Print and shaded views of the part. All mm, measured from the part's lowest x, y and z. Round coordinates to 2 decimals unless told otherwise and drop trailing zeros. Loops run counter-clockwise (first coordinate to the right, second up) from the corner with the lowest first, then second, coordinate; pieces in that order, holes last. Notation, with made-up numbers: (0.25, 46) - (59.25, 46) arc R27 cw to (59.25, 68) - close; hole circle Ø10 at (81.5, 36.5). An arc over 180 degrees is marked (long way). Use one line per item in the form item = value. Start each with the question number.
Q1. Saw through at A-A (z = 2.7). Give the cut face in (x, y), then the cut area to 3 significant figures.
Q2. Saw through at D-D (y = 4). Give the cut face in (x, z).
Q3. Saw through at B-B (x = 15.25). Give the cut face in (y, z).
Q4. Mould opens along X. For the marked faces 1 and 2 say: released by +X, released by -X, zero draft, split by the parting line, or undercut.
Q5. Saw through at C-C (y = 16). Give the cut face in (x, z), then the cut area to 3 significant figures.
Q6. Drill centre lines: line 1 (X direction, y = 10.25, z = 3.4); line 2 (X direction, y = 14, z = 1.05); line 3 (Y direction, x = 9, z = 0.5). Where is each one in solid material? Low to high.
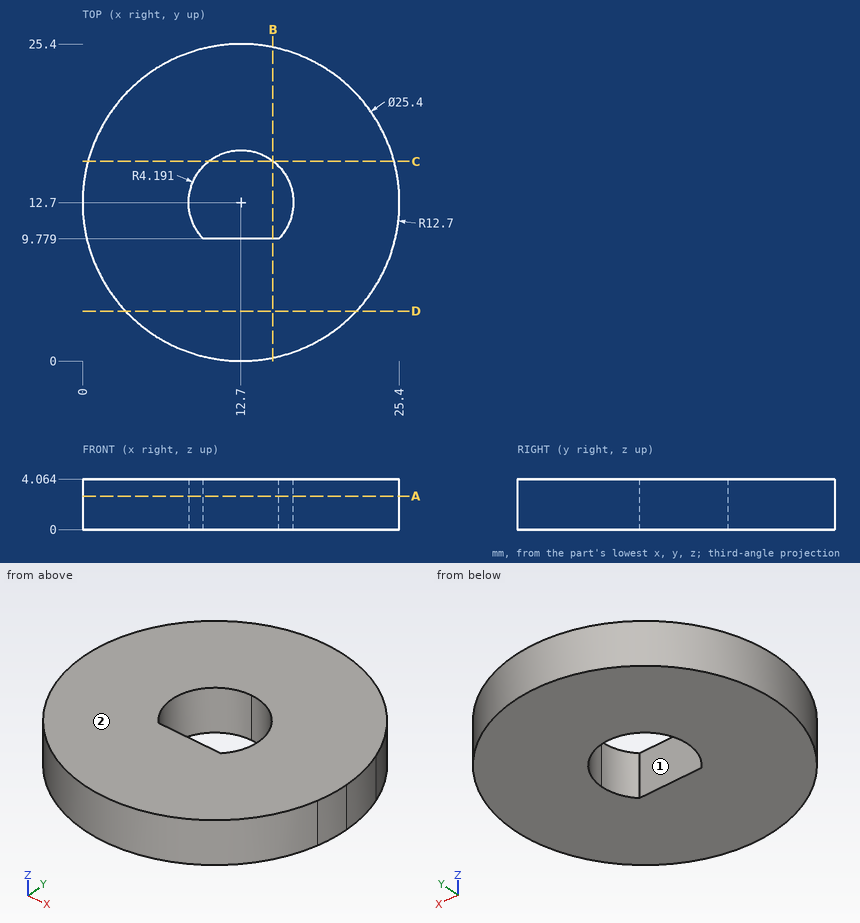
Report:
q1.outline = circle Ø25.4 at (12.7, 12.7); hole (9.69, 9.78) - (15.71, 9.78) arc R4.19 ccw (long way) to start
q1.area = 457 mm²
q2.outline = (3.45, 0) - (21.95, 0) - (21.95, 4.06) - (3.45, 4.06) - close
q3.outline = (0.26, 0) - (9.78, 0) - (9.78, 4.06) - (0.26, 4.06) - close; (16.03, 0) - (25.14, 0) - (25.14, 4.06) - (16.03, 4.06) - close
q4.face_1 = undercut
q4.face_2 = zero draft
q5.outline = (0.44, 0) - (10.12, 0) - (10.12, 4.06) - (0.44, 4.06) - close; (15.28, 0) - (24.96, 0) - (24.96, 4.06) - (15.28, 4.06) - close
q5.area = 78.7 mm²
q6.line_1 = 0.24 to 9.3, 16.1 to 25.16
q6.line_2 = 0.07 to 8.72, 16.68 to 25.33
q6.line_3 = 0.55 to 10.73, 14.67 to 24.85
